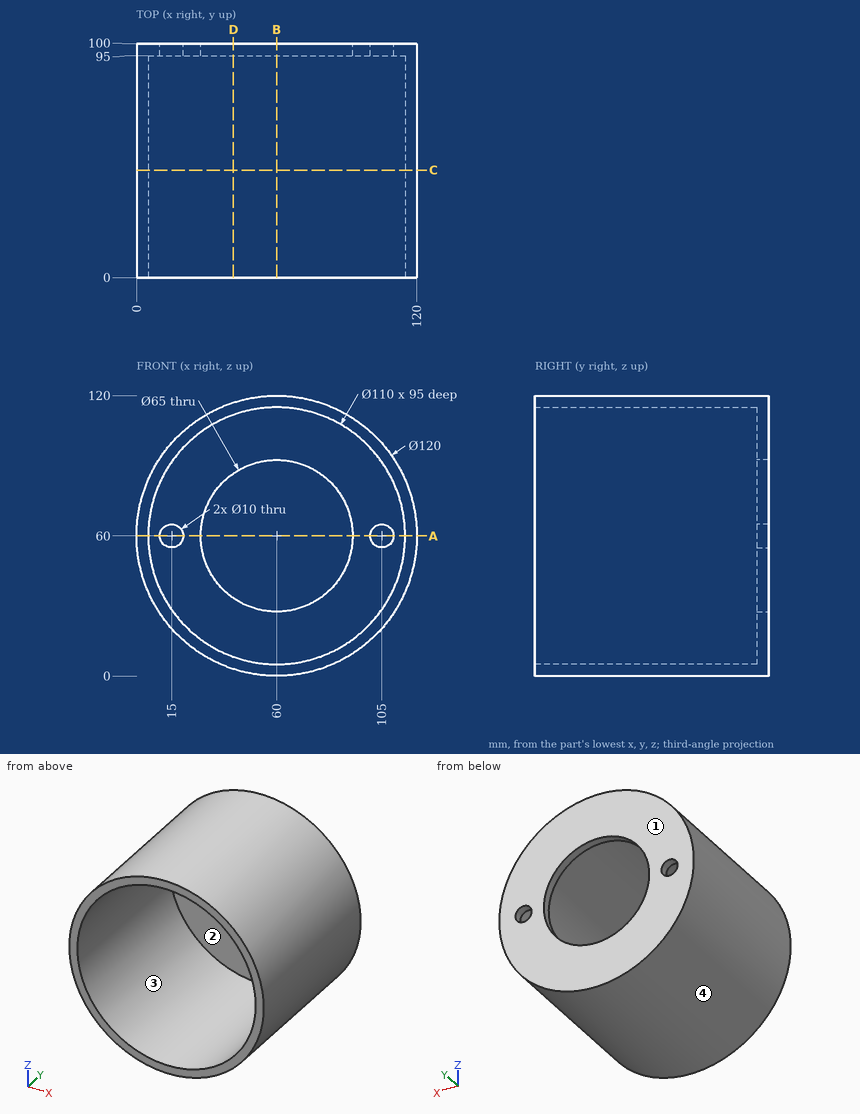
Here's the drawing with two shaded views (mm, measured from the low corner). I have some questions. Give positions to 0.01 mm unless a question says otherwise; leave off trailing zeros. Loops run counter-clockwise (first coordinate to the right, second up) from the corner with the lowest first, then second, coordinate; pieces in that order, holes last. Notation, with made-up numbers: M 18,58 L 48,58 A6 ccw 48,66 Z; hole C -37,7.25 d6. An arc over 180 degrees is marked long. Answer in a Markdown table with one row per item.
1. If I drill on line 1 along X through (y, z) = (96.3, 60); line 2 along X through (y, z) = (40, 60); line 3 along Y through (x, z) = (10, 39), over which ranges is the centre line in solid material (lowest first)?
Taken from the geometry:
| item | result |
|---|---|
| line 1 | x = 0 to 10, 20 to 27.5, 92.5 to 100, 110 to 120 |
| line 2 | x = 0 to 5, 115 to 120 |
| line 3 | y = 95 to 100 |
2. For pin 1 Ø1 at (y, z) = (12.5, 53) entering from -X; pin 2 Ø11.5 at (x, z) = (105, 60) entering from -Y; pin 3 Ø6 at (x, y) = (96.5, 85) entering from +Z, each with a flat end and sliding along its axis, tell me the tip position at first contact or that it passes through.
Taken from the geometry:
| item | result |
|---|---|
| pin 1 | stops at x = 0.35 |
| pin 2 | stops at y = 95 |
| pin 3 | stops at z = 109.78 |
3. Suppose I cut it at B-B on x = 60. Write out the boundary of the cut face in (y, z), plus the area to 4 significant figures.
Taken from the geometry:
| item | result |
|---|---|
| outline | M 0,0 L 100,0 L 100,27.5 L 95,27.5 L 95,5 L 0,5 Z; M 0,115 L 95,115 L 95,92.5 L 100,92.5 L 100,120 L 0,120 Z |
| area | 1,225 mm² |
4. Thinking about a two-plate mould opening in Z: for the marked faces 1, 2, 3 and 4, which applies, released by +Z, released by -Z, zero draft, split by the parting line, or undercut?
Taken from the geometry:
| item | result |
|---|---|
| face 1 | zero draft |
| face 2 | undercut |
| face 3 | undercut |
| face 4 | split by the parting line |
5. Suppose I cut it at C-C on y = 46. Write out the boundary of the cut face in (x, z), plus the area to 3 significant figures.
Taken from the geometry:
| item | result |
|---|---|
| outline | C 60,60 d120; hole C 60,60 d110 |
| area | 1,810 mm² |
6. Suppose I cut it at D-D on x = 41.5. Write out the boundary of the cut face in (y, z).
Taken from the geometry:
| item | result |
|---|---|
| outline | M 0,2.92 L 100,2.92 L 100,33.28 L 95,33.28 L 95,8.2 L 0,8.2 Z; M 0,111.8 L 95,111.8 L 95,86.72 L 100,86.72 L 100,117.08 L 0,117.08 Z |
7. Suppose I cut it at A-A on z = 60. Write out the boundary of the cut face in (x, y).
Taken from the geometry:
| item | result |
|---|---|
| outline | M 0,0 L 5,0 L 5,95 L 10,95 L 10,100 L 0,100 Z; M 20,95 L 27.5,95 L 27.5,100 L 20,100 Z; M 92.5,95 L 100,95 L 100,100 L 92.5,100 Z; M 110,95 L 115,95 L 115,0 L 120,0 L 120,100 L 110,100 Z |
